Design review of the part built by this model. Coordinates are the model's own, in mm. Face numbers are marked on the shaded views. Coordinates: 2 decimals unless noted, no trailing zeros. Order: outer loops, then holes, each group sorted by start corner. A loop starts at its lowest first (then second) coordinate and runs counter-clockwise, first axis right, second up.
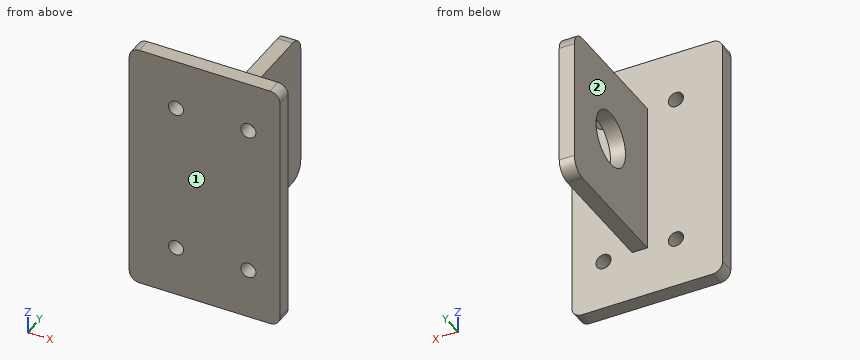
from build123d import *

# Parameters (mm, degrees)
SKETCH_1_W               = 30
SKETCH_1_H               = 50
EXTRUDE_1_DEPTH          = 3
SKETCH_2_W               = 30
SKETCH_2_H               = 30
EXTRUDE_2_DEPTH          = 3
SKETCH_3_R               = 5.45
CUT_EXTRUDE_1_DEPTH      = 3
FILLET_1_R               = 2
FILLET_2_R               = 3
SKETCH_4_R               = 1.5
CUT_EXTRUDE_2_DEPTH      = 3
MIRROR_2_COPY_1_SKETCH_R = 1.5
MIRROR_2_COPY_1_DEPTH    = 3


with BuildPart() as part:
    # 草图1 → 凸台-拉伸1 (new body)
    with BuildSketch(Plane(origin=(0, 0, 0), x_dir=(1, 0, 0), z_dir=(0, 1, 0))):
        Rectangle(SKETCH_1_W, SKETCH_1_H)
    extrude(amount=EXTRUDE_1_DEPTH)

    # 草图2 → 凸台-拉伸2 (add)
    with BuildSketch(Plane(origin=(0, 0, 0), x_dir=(0, 0, -1), z_dir=(1, 0, 0))):
        with Locations((0, 15)):
            Rectangle(SKETCH_2_W, SKETCH_2_H)
    extrude(amount=EXTRUDE_2_DEPTH)

    # 草图3 → 切除-拉伸1 (cut)
    with BuildSketch(Plane(origin=(3, 0, 0), x_dir=(0, 0, -1), z_dir=(1, 0, 0))):
        with Locations((0, 16.5)):
            Circle(SKETCH_3_R)
    extrude(amount=-CUT_EXTRUDE_1_DEPTH, mode=Mode.SUBTRACT)

    # 圆角1
    fillet_1_edges = [part.edges().sort_by_distance(p)[0] for p in [
        (-15, 1.5, -25),
        (15, 1.5, -25),
        (15, 1.5, 25),
        (-15, 1.5, 25),
    ]]
    fillet(fillet_1_edges, radius=FILLET_1_R)

    # 圆角2
    fillet_2_edges = [part.edges().sort_by_distance(p)[0] for p in [
        (1.5, 30, 15),
        (1.5, 30, -15),
    ]]
    fillet(fillet_2_edges, radius=FILLET_2_R)

    # 草图4 → 切除-拉伸2 (cut)
    with BuildSketch(Plane(origin=(0, 3, 0), x_dir=(1, 0, 0), z_dir=(0, 1, 0))):
        with Locations(Location((-5.70350483, 15, 0), (0, 0, 270))):
            Circle(SKETCH_4_R)
    cut_extrude_2 = extrude(amount=-CUT_EXTRUDE_2_DEPTH, mode=Mode.SUBTRACT)

    # 镜向1: 切除-拉伸2 across plane
    add(cut_extrude_2.mirror(Plane.XY), mode=Mode.SUBTRACT)

    # 镜向2: 切除-拉伸2 across plane
    add(cut_extrude_2.mirror(Plane(origin=(1.5, 0, 0), x_dir=(0, 0, 1), z_dir=(1, 0, 0))), mode=Mode.SUBTRACT)

    # 镜向2 copy 1 sketch → 镜向2 copy 1 (cut)
    with BuildSketch(Plane(origin=(3, 3, 0), x_dir=(-1, 0, 0), z_dir=(0, 1, 0))):
        with Locations(Location((-5.70350483, 15, 0), (0, 0, 270))):
            Circle(MIRROR_2_COPY_1_SKETCH_R)
    extrude(amount=-MIRROR_2_COPY_1_DEPTH, mode=Mode.SUBTRACT)


solid = part.part
1. Add section A-A (z = -3). Give the boundary of the cut face in (x, y), and give its area (3 significant figures).
2. Add section B-B (y = 16.5). Give the boundary of the cut face in (x, z).
3. Insertion check: pin 1 (9 mm diameter, centred on x = 3.5, z = -8, fed in from +Y); pin 2 (4 mm diameter, centred on y = 14.5, z = 6, fed in from -X); pin 3 (0.9 mm diameter, centred on x = 2, y = 11.5, fed in from +Z); pin 4 (12 mm diameter, centred on y = 10, z = 10, fed in from +X). Each pin has a flat end and moves straight along its axis. Give the tip position at first contact, or say it passes through.
4. Mouldability with a two-part tool opening along Y and no side actions: class the marked faces 1 and 2 as pulls with the +Y half, pulls with the -Y half, needs draft (parallel to the pull), parting line crosses it, or undercut.
5. Add section D-D (y = 11.75). Give the boundary of the cut face in (x, z).
6. To check wall thickness, follow line 1 (Y direction, x = 1.65, z = 0); line 2 (X direction, y = 1.6, z = 15); line 3 (Z direction, x = -6.25, y = 2.5). State the ranges of each line that lie inside material, in increasing order.
7. Add section C-C (z = 10.5). Give the boundary of the cut face in (x, y), and give its area (3 significant figures).
Solution:
1. outline: (-15, 0) - (15, 0) - (15, 3) - (3, 3) - (3, 11.95) - (0, 11.95) - (0, 3) - (-15, 3) - close; (0, 21.05) - (3, 21.05) - (3, 30) - (0, 30) - close
1. area: 144 mm2
2. outline: (0, -15) - (3, -15) - (3, -5.45) - (0, -5.45) - close; (0, 5.45) - (3, 5.45) - (3, 15) - (0, 15) - close
3. pin 1: stops at y = 30
3. pin 2: stops at x = 0
3. pin 3: stops at z = 15
3. pin 4: stops at x = 3
4. face 1: pulls with the -Y half
4. face 2: needs draft
5. outline: (0, -15) - (3, -15) - (3, -2.67) - (0, -2.67) - close; (0, 2.67) - (3, 2.67) - (3, 15) - (0, 15) - close
6. line 1: y = 0 to 11.05, 21.95 to 30
6. line 2: x = -15 to -7.2, -4.2 to 7.2, 10.2 to 15
6. line 3: z = -25 to -16.4, -13.6 to 13.6, 16.4 to 25
7. outline: (-15, 0) - (15, 0) - (15, 3) - (3, 3) - (3, 30) - (0, 30) - (0, 3) - (-15, 3) - close
7. area: 171 mm2
